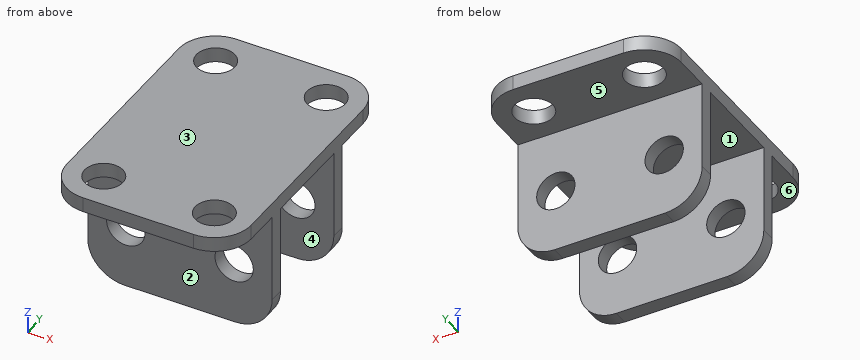
```python
from build123d import *

# Parameters (mm, degrees)
SKETCH1_W           = 25
SKETCH1_H           = 17
SKETCH1_R           = 2.6
BOSS_EXTRUDE1_DEPTH = 2
SKETCH2_W           = 25
SKETCH2_H           = 14.75
BOSS_EXTRUDE2_DEPTH = 2
SKETCH3_W           = 25
SKETCH3_H           = 2
BOSS_EXTRUDE3_DEPTH = 10
FILLET1_R           = 5
SKETCH4_R           = 2.6
CUT_EXTRUDE1_DEPTH  = 10


with BuildPart() as part:
    # Sketch1 → Boss-Extrude1 (new body)
    with BuildSketch(Plane(origin=(0, 0, 0), x_dir=(1, 0, 0), z_dir=(0, 1, 0))):
        Rectangle(SKETCH1_W, SKETCH1_H)
        with Locations((-7.345, 0)):
            Circle(SKETCH1_R, mode=Mode.SUBTRACT)
        with Locations((7.345, 0)):
            Circle(SKETCH1_R, mode=Mode.SUBTRACT)
    extrude(amount=BOSS_EXTRUDE1_DEPTH)

    # Sketch2 → Boss-Extrude2 (add)
    with BuildSketch(Plane.XY.offset(8.5)):
        with Locations((0, 7.375)):
            Rectangle(SKETCH2_W, SKETCH2_H)
    extrude(amount=BOSS_EXTRUDE2_DEPTH)

    # Mirror2: part across plane


with BuildPart() as part_1:
    add(part.part)
    add(part.part.mirror(Plane.ZX.offset(8.375)))

    # Sketch3 → Boss-Extrude3 (add)
    with BuildSketch(Plane(origin=(0, 16.75, 0), x_dir=(1, 0, 0), z_dir=(0, 1, 0))):
        with Locations((0, -9.5)):
            Rectangle(SKETCH3_W, SKETCH3_H)
    extrude(amount=BOSS_EXTRUDE3_DEPTH)

    # Mirror3: part across plane


with BuildPart() as part_2:
    add(part_1.part)
    add(part_1.part.mirror(Plane.ZX.offset(8.375)))

    # Fillet1
    fillet1_edges = [part_2.edges().sort_by_distance(p)[0] for p in [
        (12.5, 15.75, -8.5),
        (-12.5, 15.75, -8.5),
        (-12.5, 26.75, 9.5),
        (12.5, 26.75, 9.5),
        (-12.5, 1, -8.5),
        (12.5, 1, -8.5),
        (-12.5, -10, 9.5),
        (12.5, -10, 9.5),
    ]]
    fillet(fillet1_edges, radius=FILLET1_R)

    # Sketch4 → Cut-Extrude1 (cut)
    with BuildSketch(Plane(origin=(0, 0, 8.5), x_dir=(-1, 0, 0), z_dir=(0, 0, -1))):
        with Locations((-7.5, 21.75)):
            Circle(SKETCH4_R)
        with Locations((7.5, 21.75)):
            Circle(SKETCH4_R)
        with Locations((7.5, -5)):
            Circle(SKETCH4_R)
        with Locations((-7.5, -5)):
            Circle(SKETCH4_R)
    extrude(amount=-CUT_EXTRUDE1_DEPTH, mode=Mode.SUBTRACT)


solid = part_2.part
```
For this review, take the finished solid that the model builds, in its own axes (mm). Face numbers are marked on the shaded views. A direction names the side the tool comes from. Give positions to 0.01 mm unless a question says otherwise; leave off trailing zeros. Order: outer loops, then holes, each group sorted by start corner. A loop starts at its lowest first (then second) coordinate and runs counter-clockwise, first axis right, second up.
1) Take a section at D-D (z = -4). Give the boundary of the cut face in (x, y).
2) The part is to be moulded in two halves that separate along Y. For the marked faces 1, 2 and 3, say which applies: released by +Y, released by -Y, zero draft, split by the parting line, or undercut.
3) For the marked faces 4, 5 and 6, list the 3-axis set-ups (+Z, -Z, +X, -X, +Y, -Y) from which the entire face can be reached by the end or side of a thin tool; tool diameter is ignored.
4) Insertion check: pin 1 (8.5 mm diameter, centred on x = -7.5, y = 21.75, fed in from -Z); pin 2 (5 mm diameter, centred on x = 4, z = -2.5, fed in from -Y); pin 3 (3 mm diameter, centred on x = -7.345, z = 0, fed in from +Y); pin 4 (8.5 mm diameter, centred on x = -6, z = -0.5, fed in from +Y). Each pin has a flat end and moves straight along its axis. Give the tip position at first contact, or say it passes through.
5) Take a section at C-C (y = 21). Give the boundary of the cut face in (x, z).
6) Take a section at A-A (z = 0). Give the boundary of the cut face in (x, y) (3 decimals), then the cut area to 3 significant figures.
7) Take a section at B-B (x = -7). Give the boundary of the cut face in (y, z), then the cut area to 3 significant figures.
8) Wall thickness on line 1 (Y direction, x = -7.5, z = 9.55); line 2 (Y direction, x = 8, z = 5); line 3 (Z direction, x = 7, y = 8): over which ranges is each line inside the solid? List them lowest first.
Derived:
1. outline: (-12.47, 0) - (12.47, 0) - (12.47, 2) - (-12.47, 2) - close; (-12.47, 14.75) - (12.47, 14.75) - (12.47, 16.75) - (-12.47, 16.75) - close
2. face 1: undercut
2. face 2: released by -Y
2. face 3: zero draft
3. face 4: -Z, +X, -X
3. face 5: -Z, +X, -X, +Y
3. face 6: -Z, +X, -X, -Y
4. pin 1: stops at z = 8.5
4. pin 2: stops at y = 0
4. pin 3: passes through
4. pin 4: stops at y = 16.75
5. outline: (-12.5, 8.5) - (-9.99, 8.5) - (-9.99, 10.5) - (-12.5, 10.5) - close; (-5.01, 8.5) - (5.01, 8.5) - (5.01, 10.5) - (-5.01, 10.5) - close; (9.99, 8.5) - (12.5, 8.5) - (12.5, 10.5) - (9.99, 10.5) - close
6. outline: (-12.5, 0) - (-9.945, 0) - (-9.945, 2) - (-12.5, 2) - close; (-12.5, 14.75) - (-9.945, 14.75) - (-9.945, 16.75) - (-12.5, 16.75) - close; (-4.745, 0) - (4.745, 0) - (4.745, 2) - (-4.745, 2) - close; (-4.745, 14.75) - (4.745, 14.75) - (4.745, 16.75) - (-4.745, 16.75) - close; (9.945, 0) - (12.5, 0) - (12.5, 2) - (9.945, 2) - close; (9.945, 14.75) - (12.5, 14.75) - (12.5, 16.75) - (9.945, 16.75) - close
6. area: 58.4 mm2
7. outline: (-10, 8.5) - (-7.55, 8.5) - (-7.55, 10.5) - (-10, 10.5) - close; (-2.45, 8.5) - (0, 8.5) - (0, 2.58) - (2, 2.58) - (2, 8.5) - (14.75, 8.5) - (14.75, 2.58) - (16.75, 2.58) - (16.75, 8.5) - (19.2, 8.5) - (19.2, 10.5) - (-2.45, 10.5) - close; (0, -8.5) - (2, -8.5) - (2, -2.58) - (0, -2.58) - close; (14.75, -8.5) - (16.75, -8.5) - (16.75, -2.58) - (14.75, -2.58) - close; (24.3, 8.5) - (26.75, 8.5) - (26.75, 10.5) - (24.3, 10.5) - close
7. area: 100 mm2
8. line 1: y = -10 to -7.6, -2.4 to 19.15, 24.35 to 26.75
8. line 2: y = 0 to 2, 14.75 to 16.75
8. line 3: z = 8.5 to 10.5
